Geometry: final body of the model. Coordinates: model frame, mm. Face numbers are marked on the shaded views. A direction names the side the tool comes from. Give positions to 0.01 mm unless a question says otherwise; leave off trailing zeros. Order: outer loops, then holes, each group sorted by start corner. A loop starts at its lowest first (then second) coordinate and runs counter-clockwise, first axis right, second up. Notation, with made-up numbers: (68, 13.5) -> (73, 13.5) arc R24 cw to (73, 48.5) -> close; hole circle Ø4 at (19, -40). An arc over 180 degrees is marked (long way). One line per question, with ' | ' between items.
from build123d import *

# Parameters (mm, degrees)
SKETCH_1_W      = 10
SKETCH_1_H      = 10
SKETCH_1_W_2    = 8
SKETCH_1_H_2    = 8
EXTRUDE_1_DEPTH = 70


with BuildPart() as part:
    # 草图1 → 凸台-拉伸1 (new body)
    with BuildSketch(Plane.XZ.offset(70)):
        Rectangle(SKETCH_1_W, SKETCH_1_H)
        Rectangle(SKETCH_1_W_2, SKETCH_1_H_2, mode=Mode.SUBTRACT)
    extrude(amount=-EXTRUDE_1_DEPTH)


solid = part.part
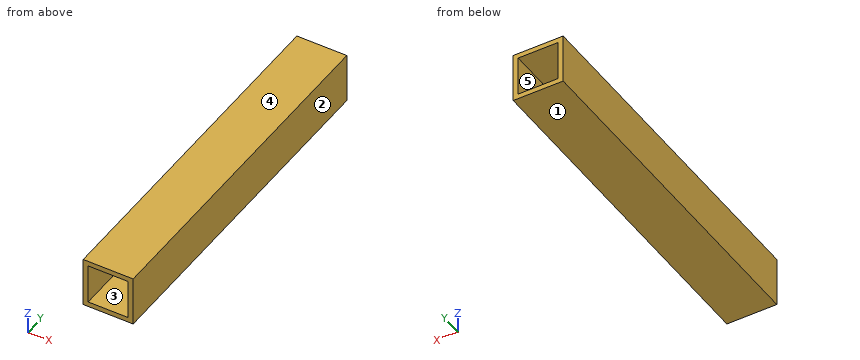
1) Set-up query: the marked faces 4 and 5. Return all of +Z, -Z, +X, -X, +Y, -Y with unobstructed straight access to the full face (end or side cutting, diameter ignored); none if empty.
Check result:
face 4: +Z, +X, -X, +Y, -Y | face 5: +Y, -Y
2) Section A-A on x = 2.75. Return loops of the section in (y, z), plus the area to 3 significant figures.
Check result:
outline: (-70, -5) -> (0, -5) -> (0, -4) -> (-70, -4) -> close; (-70, 4) -> (0, 4) -> (0, 5) -> (-70, 5) -> close | area: 140 mm^2
3) Section B-B on z = 3.25. Return loops of the section in (x, y).
Check result:
outline: (-5, -70) -> (-4, -70) -> (-4, 0) -> (-5, 0) -> close; (4, -70) -> (5, -70) -> (5, 0) -> (4, 0) -> close
4) Material intervals for probe 1 along X at (y, z) = (-8, -3.75), sorted ascending. Write a range as from..to.
Check result:
probe 1: x = -5..-4, 4..5
5) Section C-C on y = -21.5. Return loops of the section in (x, z).
Check result:
outline: (-5, -5) -> (5, -5) -> (5, 5) -> (-5, 5) -> close; hole (-4, -4) -> (4, -4) -> (4, 4) -> (-4, 4) -> close
6) Contact query for flat-ended pins moving along their axis: pin 1 Ø1.5 at (x, z) = (0, 2) entering from -Y; pin 2 Ø3 at (x, z) = (3, 0) entering from +Y. Output: stop coordinate, or through.
Check result:
pin 1: passes through | pin 2: stops at y = 0
7) Pull-direction query (X, two-part tool) for the marked faces 1, 2 and 3; classes: +X half, -X half, draft (parallel to the pull), parting line (faces both ways), or undercut.
Check result:
face 1: draft | face 2: +X half | face 3: undercut
